Autodesk Inventor part; units mm, degrees
ref_plane "YZ Plane" through (0, 0, 0) normal (1, 0, 0) x (0, 1, 0)
ref_plane "XZ Plane" through (0, 0, 0) normal (0, 1, 0) x (-1, 0, 0)
ref_plane "XY Plane" through (0, 0, 0) normal (0, 0, 1) x (1, 0, 0)
sketch "Sketch1" plane through (0, 0, 0) normal (1, 0, 0) x (0, 1, 0)
  line L0 (31.75, 0) -> (31.75, -31.75)
  line L1 (31.75, -31.75) -> (0, -31.75)
  line L2 (0, -31.75) -> (0, 0)
  line L3 (25.4, 0) -> (25.4, -6.35)
  line L4 (25.4, -6.35) -> (6.35, -6.35)
  line L5 (6.35, -6.35) -> (6.35, 0)
  line L6 (6.35, -31.75) -> (25.4, -31.75)
  line L7 (0, 0) -> (6.35, 0)
  line L8 (25.4, 0) -> (31.75, 0)
  line L9 (6.35, -19.05) -> (25.4, -19.05)
  line L10 (25.4, -19.05) -> (25.4, -25.4)
  line L11 (25.4, -25.4) -> (6.35, -25.4)
  line L12 (6.35, -25.4) -> (6.35, -19.05)
  dimension "d6" = 6.35
  dimension "d8" = 19.05
  dimension "d9" = 6.35
  dimension "d10" = 6.35
  dimension "d11" = 6.35
  dimension "d19" = 31.75
  dimension "d20" = 31.75
extrude "Extrusion1" add sketch "Sketch1" along normal blind 6.35
sketch "Sketch2" plane through (6.35, 0, 0) normal (1, 0, 0) x (0, 0, -1)
  line L0 (19.05, 25.4) -> (25.4, 25.4)
  line L1 (25.4, 25.4) -> (25.4, 6.35)
  line L2 (25.4, 6.35) -> (19.05, 6.35)
  line L3 (19.05, 6.35) -> (19.05, 25.4)
  line L4 (0, 0) -> (31.75, 0)
  line L5 (31.75, 0) -> (31.75, 31.75)
  line L6 (31.75, 31.75) -> (0, 31.75)
  line L7 (0, 31.75) -> (0, 25.4)
  line L8 (0, 25.4) -> (6.35, 25.4)
  line L9 (6.35, 25.4) -> (6.35, 6.35)
  line L10 (6.35, 6.35) -> (0, 6.35)
  line L11 (0, 6.35) -> (0, 0)
  circle A0 centre (12.7, 15.875) radius 4.7625
  dimension "d14" = 9.525
  dimension "d15" = 15.875
  dimension "d16" = 6.35
extrude "Extrusion2" cut sketch "Sketch2" against normal blind 3.175 contours A0
sketch "Sketch3" plane through (0, 25.4, 0) normal (0, 0, 1) x (1, 0, 0)
  line L0 (0, 6.35) -> (0, 0)
  line L1 (0, 0) -> (6.35, 0)
  line L2 (6.35, 6.35) -> (6.35, 0)
  line L3 (0, 6.35) -> (6.35, 6.35)
  line L4 (0, -19.05) -> (0, -25.4)
  line L5 (0, -25.4) -> (6.35, -25.4)
  line L6 (6.35, -19.05) -> (6.35, -25.4)
  line L7 (0, -19.05) -> (6.35, -19.05)
  line L8 (0, 6.35) -> (19.05, 6.35)
  line L9 (19.05, 6.35) -> (19.05, 0)
  line L10 (19.05, 0) -> (0, 0)
  line L11 (0, 0) -> (0, 6.35)
  line L12 (0, -25.4) -> (19.05, -25.4)
  line L13 (19.05, -25.4) -> (19.05, -19.05)
  line L14 (19.05, -19.05) -> (0, -19.05)
  line L15 (0, -19.05) -> (0, -25.4)
  circle A0 centre (15.875, 3.175) radius 2.159
  circle A1 centre (15.875, -22.225) radius 2.159
  dimension "d21" = 19.05
  dimension "d22" = 4.318
  dimension "d23" = 3.175
  dimension "d24" = 4.318
extrude "Extrusion3" add sketch "Sketch3" against normal blind 6.35 contours L8 L9 L10 L2 | L14 L13 L12 L6
equation "\"d20\" = d19"
properties part number "TensionerPlate"
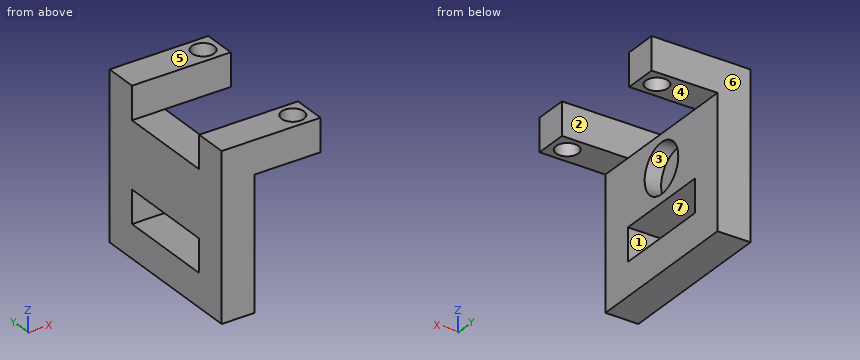
CAD build for the part. Positions are in the model's coordinates, mm. Face numbers are marked on the shaded views. A direction names the side the tool comes from. Round coordinates to 2 decimals unless told otherwise and drop trailing zeros. Order: outer loops, then holes, each group sorted by start corner. A loop starts at its lowest first (then second) coordinate and runs counter-clockwise, first axis right, second up. Notation, with made-up numbers: (-36, 10) - (17, 10) arc R17 cw to (17, 28) - close; hole circle Ø11 at (-10, -37). An arc over 180 degrees is marked (long way). Return JSON: item names as keys, results as strings.
(1) Cut at A-A (x = 7.5). Give the cut face in (y, z), then the cut area to 3 significant figures.
Answer key:
{"outline": "(0, -6.35) - (6.35, -6.35) - (6.35, 0) - (0, 0) - close; (25.4, -6.35) - (31.75, -6.35) - (31.75, 0) - (25.4, 0) - close", "area": "80.6 mm^2"}
(2) Cut at B-B (z = -20). Give the cut face in (x, y), then the cut area to 3 significant figures.
Answer key:
{"outline": "(0, 0) - (6.35, 0) - (6.35, 6.35) - (0, 6.35) - close; (0, 25.4) - (6.35, 25.4) - (6.35, 31.75) - (0, 31.75) - close", "area": "80.6 mm^2"}
(3) Tool access for the marked faces 1, 2 and 3: list every direction of +Z, -Z, +X, -X, +Y, -Y with a clear straight run to the whole face (end or side of a thin tool).
Answer key:
{"face 1": "+X, -X", "face 2": "+Z, +X, -X", "face 3": "+X"}
(4) Pin check, flat tips, straight feed: pin 1 Ø5 at (y, z) = (15, -20.5) entering from +X; pin 2 Ø3 at (x, y) = (14, 2) entering from -Z; pin 3 Ø3 at (x, y) = (2, 17.5) entering from +Z. Stop position of each tip, or through.
Answer key:
{"pin 1": "stops at x = 6.35", "pin 2": "stops at z = -6.35", "pin 3": "stops at z = -6.35"}
(5) Wall check: probe 1 along Y at (x, z) = (2, -4); probe 2 along Y at (x, z) = (4.3, -12.7); probe 3 along Z at (x, y) = (1.75, 14.5). Give the ranges that are in metal, low to high. Write a range as from..to.
Answer key:
{"probe 1": "y = 0..6.35, 25.4..31.75", "probe 2": "y = 0..11.11, 20.64..31.75", "probe 3": "z = -31.75..-25.4, -19.05..-6.35"}
(6) Pull direction Z, two halves, no side cores. Call the marked faces 4, 5, 6 and 7: +Z half, -Z half, draft (parallel to the pull), parting line (faces both ways), or undercut.
Answer key:
{"face 4": "-Z half", "face 5": "+Z half", "face 6": "draft", "face 7": "undercut"}
